For this review, take the finished solid that the model builds, in its own axes (mm). A direction names the side the tool comes from. Round coordinates to 2 decimals unless told otherwise and drop trailing zeros. Write each loop counter-clockwise with the first axis right and the second up, starting at its lowest first coordinate (ties: lowest second). Pieces come first, ordered by that corner, then holes. Notation, with made-up numbers: (63, 3) -> (104, 3) arc R11 ccw to (104, 11) -> close; hole circle Ø7 at (-7, 23.5). An arc over 180 degrees is marked (long way). Write each question's results on one line, items separated by ' | '. Start each with the question number.
Item 1: Clearance check with flat-ended pins moving along their axes: pin 1 (1.7 mm diameter, centred on x = 1.5, z = 0.5, fed in from +Y); pin 2 (1.5 mm diameter, centred on x = 3, y = 3, fed in from -Z); pin 3 (2 mm diameter, centred on x = 0.5, y = 3.5, fed in from -Z). State where each tip first meets the part, or that it passes through.
Item 2: Add section D-D (y = -0.25). State the section outline as (x, z) points.
Item 3: Add section C-C (x = 3.7). State the section outline as (y, z) points, plus the area to 3 significant figures.
Item 4: Add section A-A (z = 0). State the section outline as (x, y) points, plus the area to 3 significant figures.
Item 5: Add section B-B (y = 4.75). State the section outline as (x, z) points.
Item 6: Tool access review of faces 4 (the flat face through (2.028, 1.175, -5.111)), 5 (the flat face through (2.03, 1.03, 4.26)), 6 (the flat face through (2.028, 4.145, -3.338)): name each direction out of +Z, -Z, +X, -X, +Y, -Y from which nothing blocks a thin tool from reaching the whole face with its end or side.
Item 7: The part is to be moulded in two halves that separate along Z. For faces 1 (the flat face through (2, 3, 0)), 2 (the flat face through (0, 2.5, -0.9)), 3 (the flat face through (2.03, 0.52, 6.99)), say which applies: +Z half, -Z half, draft (parallel to the pull), parting line (faces both ways), or undercut.
Item 8: To check wall thickness, follow line 1 along Y through (x, z) = (1.05, 0); line 2 along Z through (x, y) = (2.8, 1.25); line 3 along Z through (x, y) = (2.3, 5.25). State the ranges of each line that lie inside material, in increasing order.
from build123d import *

# Parameters (mm, degrees)
CROQUIS1_R              = 2.1
SALIENTE_EXTRUIR1_DEPTH = 4
SALIENTE_EXTRUIR2_DEPTH = 4
SALIENTE_EXTRUIR3_DEPTH = 4
SALIENTE_EXTRUIR4_DEPTH = 4
REDONDEO1_R             = 1.2


with BuildPart() as part:
    # Croquis1 → Saliente-Extruir1 (new body)
    with BuildSketch(Plane(origin=(0, 0, 0), x_dir=(0, 0, -1), z_dir=(1, 0, 0))):
        Polygon((3.464101615, 0), (1.732050808, 3), (-1.732050808, 3), (-3.464101615, 0), (-1.732050808, -3), (1.732050808, -3), align=None)
        Circle(CROQUIS1_R, mode=Mode.SUBTRACT)
    extrude(amount=SALIENTE_EXTRUIR1_DEPTH)

    # Croquis2 → Saliente-Extruir2 (add, through all)
    with BuildSketch(Plane(origin=(4, 0, 0), x_dir=(0, 0, -1), z_dir=(1, 0, 0))):
        Polygon((6.990847349, 2.515265858), (3.464101615, 0), (1.732050808, 3), (4.988660177, 5.322605307), align=None)
    extrude(amount=-SALIENTE_EXTRUIR2_DEPTH)

    # Croquis12 → Saliente-Extruir3 (add, through all)
    with BuildSketch(Plane(origin=(4, 0, 0), x_dir=(0, 0, -1), z_dir=(1, 0, 0))):
        Polygon((-7.281299997, 6.043148081), (-1.732050808, 3), (-3.464101615, 0), (-5.080008932, 2.097632781), (-5.736212746, -0.706387852), (-8.278793458, 1.780764673), align=None)
    extrude(amount=-SALIENTE_EXTRUIR3_DEPTH)

    # Croquis13 → Saliente-Extruir4 (add, through all)
    with BuildSketch(Plane(origin=(4, 0, 0), x_dir=(0, 0, -1), z_dir=(1, 0, 0))):
        Polygon((6.990847349, 2.515265858), (9.278705783, 7.966164247), (6.097551134, 9.301362773), (4.988660177, 5.322605307), align=None)
    extrude(amount=-SALIENTE_EXTRUIR4_DEPTH)

    # Redondeo1
    redondeo1_edges = [part.edges().sort_by_distance(p)[0] for p in [
        (2, 2.515265858, -6.990847349),
        (2, 9.301362773, -6.097551134),
        (2, 7.966164247, -9.278705783),
    ]]
    fillet(redondeo1_edges, radius=REDONDEO1_R)


solid = part.part
Responses:
1) pin 1: stops at y = 3 | pin 2: stops at z = -7.51 | pin 3: stops at z = -7.82
2) outline: (0, -3.32) -> (4, -3.32) -> (4, -2.09) -> (0, -2.09) -> close; (0, 2.09) -> (4, 2.09) -> (4, 3.32) -> (0, 3.32) -> close; (0, 5.63) -> (4, 5.63) -> (4, 6.2) -> (0, 6.2) -> close
3) outline: (-3, -1.73) -> (0, -3.46) -> (2.32, -6.71) arc R1.2 ccw to (2.83, -7.12) -> (6.86, -8.81) arc R1.2 ccw to (8.43, -8.17) -> (8.77, -7.35) arc R1.2 ccw to (7.99, -5.73) -> (5.32, -4.99) -> (3, -1.73) -> (3, 1.73) -> (6.04, 7.28) -> (1.78, 8.28) -> (-0.71, 5.74) -> (2.1, 5.08) -> (0, 3.46) -> (-3, 1.73) -> close; hole circle Ø4.2 at (0, 0) | area: 69.6 mm^2
4) outline: (0, -3) -> (4, -3) -> (4, -2.1) -> (0, -2.1) -> close; (0, 2.1) -> (4, 2.1) -> (4, 3) -> (0, 3) -> close | area: 7.20 mm^2
5) outline: (0, -7.93) -> (4, -7.93) -> (4, -4.19) -> (0, -4.19) -> close; (0, 4.92) -> (4, 4.92) -> (4, 7.58) -> (0, 7.58) -> close
6) face 4: -Z, +X, -X, -Y | face 5: +X, -X, -Y | face 6: +X, -X, +Y
7) face 1: undercut | face 2: draft | face 3: +Z half
8) line 1: y = -3 to -2.1, 2.1 to 3 | line 2: z = -5.22 to -1.69, 1.69 to 4.43, 5.28 to 7.74 | line 3: z = -8.14 to -4.89, 5.83 to 7.47
